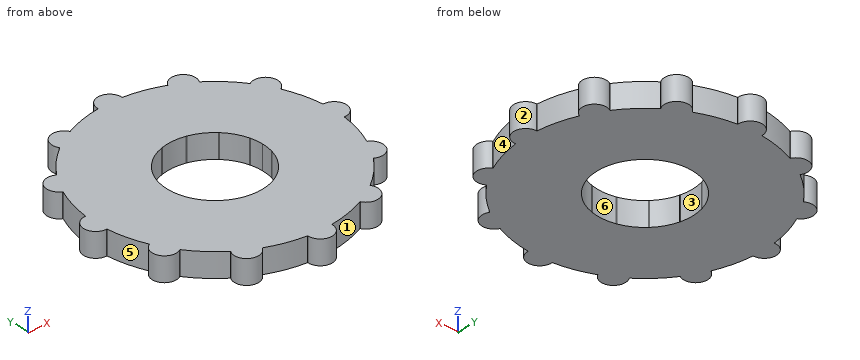
from build123d import *

# Parameters (mm, degrees)
BOSS_EXTRUDE1_DEPTH = 10


with BuildPart() as part:
    # Sketch1 → Boss-Extrude1 (new body)
    with BuildSketch(Plane.XY):
        with BuildLine():
            Line((-5.055544828, 50), (-5.055544828, 49.743758066))
            ThreePointArc((-5.055544828, 49.743758066), (-12.940952255, 48.296291315), (-20.493648782, 45.607130579))
            Line((-20.493648782, 45.607130579), (-20.621769749, 45.829042603))
            ThreePointArc((-20.621769749, 45.829042603), (-27.527772414, 47.67950044), (-29.378230251, 40.773497775))
            Line((-29.378230251, 40.773497775), (-29.250109284, 40.551585751))
            ThreePointArc((-29.250109284, 40.551585751), (-35.355339059, 35.355339059), (-40.551585751, 29.250109284))
            Line((-40.551585751, 29.250109284), (-40.773497775, 29.378230251))
            ThreePointArc((-40.773497775, 29.378230251), (-47.67950044, 27.527772414), (-45.829042603, 20.621769749))
            Line((-45.829042603, 20.621769749), (-45.607130579, 20.493648782))
            ThreePointArc((-45.607130579, 20.493648782), (-48.296291315, 12.940952255), (-49.743758066, 5.055544828))
            Line((-49.743758066, 5.055544828), (-50, 5.055544828))
            ThreePointArc((-50, 5.055544828), (-55.055544828, 0), (-50, -5.055544828))
            Line((-50, -5.055544828), (-49.743758066, -5.055544828))
            ThreePointArc((-49.743758066, -5.055544828), (-48.296291315, -12.940952255), (-45.607130579, -20.493648782))
            Line((-45.607130579, -20.493648782), (-45.829042603, -20.621769749))
            ThreePointArc((-45.829042603, -20.621769749), (-47.67950044, -27.527772414), (-40.773497775, -29.378230251))
            Line((-40.773497775, -29.378230251), (-40.551585751, -29.250109284))
            ThreePointArc((-40.551585751, -29.250109284), (-35.355339059, -35.355339059), (-29.250109284, -40.551585751))
            Line((-29.250109284, -40.551585751), (-29.378230251, -40.773497775))
            ThreePointArc((-29.378230251, -40.773497775), (-27.527772414, -47.67950044), (-20.621769749, -45.829042603))
            Line((-20.621769749, -45.829042603), (-20.493648782, -45.607130579))
            ThreePointArc((-20.493648782, -45.607130579), (-12.940952255, -48.296291315), (-5.055544828, -49.743758066))
            Line((-5.055544828, -49.743758066), (-5.055544828, -50))
            ThreePointArc((-5.055544828, -50), (0, -55.055544828), (5.055544828, -50))
            Line((5.055544828, -50), (5.055544828, -49.743758066))
            ThreePointArc((5.055544828, -49.743758066), (12.940952255, -48.296291315), (20.493648782, -45.607130579))
            Line((20.493648782, -45.607130579), (20.621769749, -45.829042603))
            ThreePointArc((20.621769749, -45.829042603), (27.527772414, -47.67950044), (29.378230251, -40.773497775))
            Line((29.378230251, -40.773497775), (29.250109284, -40.551585751))
            ThreePointArc((29.250109284, -40.551585751), (35.355339059, -35.355339059), (40.551585751, -29.250109284))
            Line((40.551585751, -29.250109284), (40.773497775, -29.378230251))
            ThreePointArc((40.773497775, -29.378230251), (47.67950044, -27.527772414), (45.829042603, -20.621769749))
            Line((45.829042603, -20.621769749), (45.607130579, -20.493648782))
            ThreePointArc((45.607130579, -20.493648782), (48.296291315, -12.940952255), (49.743758066, -5.055544828))
            Line((49.743758066, -5.055544828), (50, -5.055544828))
            ThreePointArc((50, -5.055544828), (55.055544828, 0), (50, 5.055544828))
            Line((50, 5.055544828), (49.743758066, 5.055544828))
            ThreePointArc((49.743758066, 5.055544828), (48.296291315, 12.940952255), (45.607130579, 20.493648782))
            Line((45.607130579, 20.493648782), (45.829042603, 20.621769749))
            ThreePointArc((45.829042603, 20.621769749), (47.67950044, 27.527772414), (40.773497775, 29.378230251))
            Line((40.773497775, 29.378230251), (40.551585751, 29.250109284))
            ThreePointArc((40.551585751, 29.250109284), (35.355339059, 35.355339059), (29.250109284, 40.551585751))
            Line((29.250109284, 40.551585751), (29.378230251, 40.773497775))
            ThreePointArc((29.378230251, 40.773497775), (27.527772414, 47.67950044), (20.621769749, 45.829042603))
            Line((20.621769749, 45.829042603), (20.493648782, 45.607130579))
            ThreePointArc((20.493648782, 45.607130579), (12.940952255, 48.296291315), (5.055544828, 49.743758066))
            Line((5.055544828, 49.743758066), (5.055544828, 50))
            ThreePointArc((5.055544828, 50), (0, 55.055544828), (-5.055544828, 50))
        make_face()
        with BuildLine():
            ThreePointArc((-19.274651306, -5.337397964), (-19.565972123, -5.470493987), (-19.84828049, -5.621769749))
            Line((-19.84828049, -5.621769749), (-19.285788402, -5.297014791))
            ThreePointArc((-19.285788402, -5.297014791), (-19.323926995, -5.156146381), (-19.361036662, -5.015003426))
            ThreePointArc((-19.361036662, -5.015003426), (-20, 0), (-19.361036662, 5.015003426))
            ThreePointArc((-19.361036662, 5.015003426), (-19.318516526, 5.176380902), (-19.274651306, 5.337397964))
            ThreePointArc((-19.274651306, 5.337397964), (-17.320508076, 10), (-14.25964788, 14.023638698))
            ThreePointArc((-14.25964788, 14.023638698), (-14.142135624, 14.142135624), (-14.023638698, 14.25964788))
            ThreePointArc((-14.023638698, 14.25964788), (-10, 17.320508076), (-5.337397964, 19.274651306))
            ThreePointArc((-5.337397964, 19.274651306), (-5.176380902, 19.318516526), (-5.015003426, 19.361036662))
            ThreePointArc((-5.015003426, 19.361036662), (0, 20), (5.015003426, 19.361036662))
            ThreePointArc((5.015003426, 19.361036662), (5.176380902, 19.318516526), (5.337397964, 19.274651306))
            ThreePointArc((5.337397964, 19.274651306), (10, 17.320508076), (14.023638698, 14.25964788))
            ThreePointArc((14.023638698, 14.25964788), (14.142135624, 14.142135624), (14.25964788, 14.023638698))
            ThreePointArc((14.25964788, 14.023638698), (17.320508076, 10), (19.274651306, 5.337397964))
            ThreePointArc((19.274651306, 5.337397964), (19.318516526, 5.176380902), (19.361036662, 5.015003426))
            ThreePointArc((19.361036662, 5.015003426), (19.839616091, 2.527772414), (20, 0))
            ThreePointArc((20, 0), (19.839616091, -2.527772414), (19.361036662, -5.015003426))
            ThreePointArc((19.361036662, -5.015003426), (19.318516526, -5.176380902), (19.274651306, -5.337397964))
            ThreePointArc((19.274651306, -5.337397964), (17.320508076, -10), (14.25964788, -14.023638698))
            ThreePointArc((14.25964788, -14.023638698), (14.142135624, -14.142135624), (14.023638698, -14.25964788))
            ThreePointArc((14.023638698, -14.25964788), (10, -17.320508076), (5.337397964, -19.274651306))
            ThreePointArc((5.337397964, -19.274651306), (5.176380902, -19.318516526), (5.015003426, -19.361036662))
            ThreePointArc((5.015003426, -19.361036662), (0, -20), (-5.015003426, -19.361036662))
            ThreePointArc((-5.015003426, -19.361036662), (-5.176380902, -19.318516526), (-5.337397964, -19.274651306))
            ThreePointArc((-5.337397964, -19.274651306), (-10, -17.320508076), (-14.023638698, -14.25964788))
            ThreePointArc((-14.023638698, -14.25964788), (-14.142135624, -14.142135624), (-14.25964788, -14.023638698))
            ThreePointArc((-14.25964788, -14.023638698), (-17.320508076, -10), (-19.274651306, -5.337397964))
        make_face(mode=Mode.SUBTRACT)
    extrude(amount=BOSS_EXTRUDE1_DEPTH)


solid = part.part
Input: part model. Units: mm. Frame: model coordinates. Face numbers are marked on the shaded views. A direction names the side the tool comes from. Coordinates: 2 decimals unless noted, no trailing zeros. Loops run counter-clockwise (first coordinate to the right, second up) from the corner with the lowest first, then second, coordinate; pieces in that order, holes last.
(1) Section A-A on x = 0. Return the cut outline in (y, z).
(2) Material intervals for probe 1 along X at (y, z) = (46, 4.25); probe 2 along Y at (x, z) = (-7.5, 5.25); probe 3 along Y at (x, z) = (9, 3), sorted ascending.
(3) First-contact query: pin 1 Ø1.5 at (y, z) = (4, 2.5) entering from -X; pin 2 Ø1.5 at (x, z) = (27, 3.5) entering from +Y; pin 3 Ø1.5 at (y, z) = (28, 2.5) entering from +X. Flat tips, straight axial feed; report the tip coordinate or a pass-through.
(4) Section C-C on y = -25.5. Return the cut outline in (x, z), then the cut area to 3 significant figures.
(5) Section B-B on x = -25. Return the cut outline in (y, z), then the cut area to 3 significant figures.
(6) Set-up query: the marked faces 1, 2 and 3. Return all of +Z, -Z, +X, -X, +Y, -Y with unobstructed straight access to the full face (end or side cutting, diameter ignored); none if empty.
(7) Pull-direction query (X, two-part tool) for the marked faces 4, 5 and 6; classes: released by +X, released by -X, zero draft, split by the parting line, or undercut.
Data:
1. outline: (-55.06, 0) - (-20, 0) - (-20, 10) - (-55.06, 10) - close; (20, 0) - (55.06, 0) - (55.06, 10) - (20, 10) - close
2. probe 1: x = -29.27 to -20.73, -19.6 to 19.6, 20.73 to 29.27
2. probe 2: y = -49.43 to -18.54, 18.54 to 49.43
2. probe 3: y = -49.18 to -17.86, 17.86 to 49.18
3. pin 1: stops at x = -53.87
3. pin 2: stops at y = 48.2
3. pin 3: stops at x = 47.83
4. outline: (-48.33, 0) - (48.33, 0) - (48.33, 10) - (-48.33, 10) - close
4. area: 967 mm2
5. outline: (-48.36, 0) - (48.36, 0) - (48.36, 10) - (-48.36, 10) - close
5. area: 967 mm2
6. face 1: +Z, -Z, -Y
6. face 2: +Z, -Z, +X
6. face 3: +Z, -Z
7. face 4: released by +X
7. face 5: released by -X
7. face 6: undercut
